```python
from build123d import *
from build123d.topology import SkipClean

# Parameters (mm, degrees)
SKETCH_1_R               = 10
EXTRUDE_1_DEPTH          = 30
SKETCH_2_R               = 7.05
CUT_EXTRUDE_1_DEPTH      = 20
REVOLVE_10_ANGLE         = 180
CUT_EXTRUDE_2_DEPTH      = 52.961524228
CUT_EXTRUDE_2_DEPTH_BACK = 52.961524228
EXTRUDE_2_DEPTH          = 10
CUT_EXTRUDE_START        = -2.5
CUT_EXTRUDE_3_DEPTH      = 2.5
EXTRUDE_START            = 10
SKETCH_11_R              = 10
SKETCH_11_R_2            = 7.05
EXTRUDE_3_DEPTH          = 10
HOLE_WIZARD_M2_5_1_D     = 2.9


# Read off the part's stored shape, not the designer's step: the revolve step
with BuildPart() as part:
    # Sketch 1 → Extrude 1 (new body)
    with BuildSketch(Plane(origin=(0, 0, 0), x_dir=(1, 0, 0), z_dir=(0, 1, 0))):
        with Locations(Location((0, 0, 0), (0, 0, 270))):
            Circle(SKETCH_1_R)
    extrude(amount=EXTRUDE_1_DEPTH)

    # Sketch 2 → Cut-Extrude 1 (cut)
    with BuildSketch(Plane.XZ):
        with Locations(Location((0, 0, 0), (0, 0, 270))):
            Circle(SKETCH_2_R)
    extrude(amount=-CUT_EXTRUDE_1_DEPTH, mode=Mode.SUBTRACT)



with BuildPart() as body_2:
    # Revolve 1 outline → Revolve 1 (revolve)
    with BuildSketch(Plane.XZ.offset(-40)):
        with BuildLine():
            Line((0, 1e-08), (0, -10))
            ThreePointArc((0, -10), (7.071067815, -7.071067808), (10, 1e-08))
            Line((10, 1e-08), (0, 1e-08))
        make_face()
    revolve(axis=Axis((0, 40, 0), (0, 0, 1)))

    # Sketch 5 → Cut-Revolve 3 (revolve, cut)
    with BuildSketch(Plane.XY):
        with BuildLine():
            Line((0, 45.252296995), (0, 34.747703005))
            ThreePointArc((0, 34.747703005), (5.252296995, 40), (0, 45.252296995))
        make_face()
    revolve(axis=Axis((0, 0, 0), (0, 1, 0)), mode=Mode.SUBTRACT)


with BuildPart() as part_1:
    with SkipClean():  # the faces are left unmerged after this step: merging them gives an invalid solid
        add(part.part)

        add(body_2.part)  # Revolve 10 merges body 2
        # Sketch 6 → Revolve 10 (revolve, symmetric)
        with BuildSketch(Plane(origin=(0, 0, 0), x_dir=(0, 0, -1), z_dir=(1, 0, 0))) as revolve_10_sk:
            with BuildLine():
                Line((0, 30), (0, 30.711529751))
                ThreePointArc((0, 30.711529751), (5.980054101, 33.531969517), (7.351370698, 40))
                Line((7.351370698, 40), (10, 40))
                Line((10, 40), (10, 30))
                Line((10, 30), (0, 30))
            make_face()
        revolve(axis=Axis((0, 0, 0), (0, 1, 0)), revolution_arc=REVOLVE_10_ANGLE / 2)
        revolve(revolve_10_sk.sketch, axis=Axis((0, 0, 0), (0, -1, 0)), revolution_arc=REVOLVE_10_ANGLE / 2)
    add(part_1.part.scale(1), mode=Mode.REPLACE)  # the faces are merged on a copy

    # Sketch 7 → Cut-Extrude 2 (cut, two sides: drawn at the far end of the back side and taken through both)
    with BuildSketch(Plane(origin=(0, 0, 0), x_dir=(0, 0, -1), z_dir=(1, 0, 0)).offset(-CUT_EXTRUDE_2_DEPTH_BACK)):
        with BuildLine():
            Line((-10, 24.679295292), (-17.050906842, 49.125599249))
            Line((-17.050906842, 49.125599249), (0, 49.125599249))
            Line((0, 49.125599249), (0, 34.049122638))
            ThreePointArc((0, 34.049122638), (-2.58520571, 28.084119755), (-8.705629602, 25.892098007))
            ThreePointArc((-8.705629602, 25.892098007), (-9.615626451, 25.566183836), (-10, 24.679295292))
        make_face()
    extrude(amount=CUT_EXTRUDE_2_DEPTH + CUT_EXTRUDE_2_DEPTH_BACK, mode=Mode.SUBTRACT)

    # Sketch 8 → Extrude 2 (add, symmetric)
    with BuildSketch(Plane(origin=(0, 0, 0), x_dir=(0, 0, -1), z_dir=(1, 0, 0))):
        with BuildLine():
            Line((0, 32.693889078), (0, 30))
            Line((0, 30), (-1.073327621, 30))
            ThreePointArc((-1.073327621, 30), (-0.278211386, 31.243969205), (0, 32.693889078))
        make_face()
    extrude(amount=EXTRUDE_2_DEPTH, both=True)

    # Sketch 10 → Cut-Extrude 3 (cut)
    with BuildSketch(Plane(origin=(0, 15, 0), x_dir=(1, 0, 0), z_dir=(0, 1, 0)).offset(CUT_EXTRUDE_START)):
        with BuildLine():
            Line((-8.660254038, 5), (-3.31662479, 5))
            ThreePointArc((-3.31662479, 5), (0, 6), (3.31662479, 5))
            Line((3.31662479, 5), (8.660254038, 5))
            ThreePointArc((8.660254038, 5), (0, 10), (-8.660254038, 5))
        make_face()
    extrude(amount=CUT_EXTRUDE_3_DEPTH, mode=Mode.SUBTRACT)

    # Sketch 11 → Extrude 3 (add)
    with BuildSketch(Plane.XZ.offset(EXTRUDE_START)):
        with Locations(Location((0, 0, 0), (0, 0, 270))):
            Circle(SKETCH_11_R)
        with Locations(Location((0, 0, 0), (0, 0, 270))):
            Circle(SKETCH_11_R_2, mode=Mode.SUBTRACT)
    extrude(amount=-EXTRUDE_3_DEPTH)

    # Hole Wizard M2.5 _ _1 (through all)
    with Locations(Plane.XY.offset(10)):
        with Locations((0, 2)):
            Hole(HOLE_WIZARD_M2_5_1_D / 2)


solid = part_1.part
```
Verification items for the finished model (mm, model axes). A direction names the side the tool comes from. Coordinates: 2 decimals unless noted, no trailing zeros. Loops run counter-clockwise (first coordinate to the right, second up) from the corner with the lowest first, then second, coordinate; pieces in that order, holes last. Notation, with made-up numbers: (33.5, -31) - (78.5, -31) arc R14 cw to (78.5, -16) - close; hole circle Ø7 at (-33, 42.25). An arc over 180 degrees is marked (long way). Answer as a JSON object with one key per item and string values.
(1) Go/stop test with flat-tipped pins: pin 1 Ø5 at (y, z) = (28, -5.5) entering from +X; pin 2 Ø4 at (x, z) = (-2, -1.5) entering from -Y; pin 3 Ø0.8 at (x, y) = (-7.5, 14.5) entering from -Z. Record where each tip stops, or that it passes through.
Response:
{"pin 1": "stops at x = 9.54", "pin 2": "stops at y = 20", "pin 3": "stops at z = -5"}
(2) Cross-section at C-C, the plane x = 2.25. Record the boundary of the cut face in (y, z), then the cut area to 3 significant figures.
Response:
{"outline": "(-10, -9.74) - (12.5, -9.74) - (12.5, -6.68) - (-10, -6.68) - close; (-10, 6.68) - (20, 6.68) - (20, -6.68) - (15, -6.68) - (15, -9.74) - (40, -9.74) arc R9.74 ccw to (49.74, 0) - (44.75, 0) arc R4.75 cw to (35.25, 0) - (32.69, 0) arc R3.92 cw to (30, 1.07) arc R8.17 cw to (25.89, 8.71) arc R1.22 ccw to (25.43, 9.74) - (-10, 9.74) - close", "area": "481 mm²"}
(3) Cross-section at B-B, the plane y = 2. Record the boundary of the cut face in (x, z), then the cut area to 3 significant figures.
Response:
{"outline": "(-1.45, -9.89) - (-1.45, -6.9) arc R7.05 cw to (-1.45, 6.9) - (-1.45, 9.89) arc R10 ccw to start; (1.45, -9.89) arc R10 ccw to (1.45, 9.89) - (1.45, 6.9) arc R7.05 cw to (1.45, -6.9) - close", "area": "141 mm²"}
(4) Mould release check, pull along Y, two halves, no side actions. Record for faces 1 (the flat face through (0, 20, 0)), 2 (the cylindrical face through (-0.78, 3.22, 8.43)), 3 (the cylindrical face through (0.14, 31.22, 0.29)): pulls with the +Y half, pulls with the -Y half, needs draft (parallel to the pull), parting line crosses it, or undercut.
Response:
{"face 1": "pulls with the -Y half", "face 2": "undercut", "face 3": "pulls with the +Y half"}
(5) Access from +Z, -Z, +X, -X, +Y, -Y to the whole of each face (thin tool, end or side, straight path). Record for faces 4 (the cylindrical face through (0.31, 4.79, 7.043)), 5 (the flat face through (0, 12.5, -8)), 6 (the flat face through (2.1, 45.3, 0)).
Response:
{"face 4": "-Y", "face 5": "-Z, +X, -X", "face 6": "+Z, +X, -X, +Y"}
(6) Cross-section at A-A, the plane z = -8. Record the boundary of the cut face in (x, y).
Response:
{"outline": "(-6, -10) - (6, -10) - (6, 12.5) - (-6, 12.5) - close; (-6, 15) - (6, 15) - (6, 40) arc R6 ccw to (-6, 40) - close; hole circle Ø2.9 at (0, 2)"}
(7) Scan lines: line 1 along X through (y, z) = (0.5, 0); line 2 along Y through (x, z) = (0, -8.55); line 3 along Y through (x, z) = (0, -8.35). Record each from-to range of solid material in increasing order.
Response:
{"line 1": "x = -10 to -7.05, 7.05 to 10", "line 2": "y = -10 to 0.55, 3.45 to 12.5, 15 to 45.19", "line 3": "y = -10 to 0.55, 3.45 to 12.5, 15 to 45.5"}
(8) Cross-section at D-D, the plane z = 4.5. Record the boundary of the cut face in (x, y), then the cut area to 3 significant figures.
Response:
{"outline": "(-8.93, -10) - (-5.43, -10) - (-5.43, 20) - (5.43, 20) - (5.43, -10) - (8.93, -10) - (8.93, 26.75) - (-8.93, 26.75) - close", "area": "331 mm²"}
